Build history of the part. All positions in model axes, mm. Face numbers are marked on the shaded views. A direction names the side the tool comes from. Give positions to 0.01 mm unless a question says otherwise; leave off trailing zeros. Loops run counter-clockwise (first coordinate to the right, second up) from the corner with the lowest first, then second, coordinate; pieces in that order, holes last. Notation, with made-up numbers: (7.5, 41.25) - (54.5, 41.25) arc R25 ccw to (54.5, 53.25) - close; hole circle Ø7 at (-16.75, 47). An arc over 180 degrees is marked (long way). Return JSON: item names as keys, results as strings. Group by question number.
1) Drop flat-ended pins along their axis: pin 1 (5 mm diameter, centred on x = 1, y = 46.5, fed in from +Z); pin 2 (11.5 mm diameter, centred on y = 0, z = 38.1, fed in from -X). Give the stop position or say it passes through.
2) Slice it at A-A (z = 57). List the corners of the cut face in (x, y).
3) Mould opens along Y. For the marked faces 1, 2, 3 and 4 say: released by +Y, released by -Y, zero draft, split by the parting line, or undercut.
4) Slice it at D-D (y = 0). List the corners of the cut face in (x, z) (3 decimals), and give its area (3 significant figures).
5) 3-axis set-ups, long thin cutter, end or side, ignore diameter. For the marked faces 5 and 6: which of +Z, -Z, +X, -X, +Y, -Y reach the whole face in a straight line?
6) Drill centre lines: probe 1 along X at (y, z) = (10, 58); probe 2 along Y at (x, z) = (-71, 38); probe 3 along Y at (x, z) = (-35, 23.5). Where is each one in solid material? Low to high. Write a range as from..to.
7) Slice it at B-B (y = -12.5). List the corners of the cut face in (x, z).
8) Slice it at C-C (x = 0). List the corners of the cut face in (y, z), and give its area (3 significant figures).
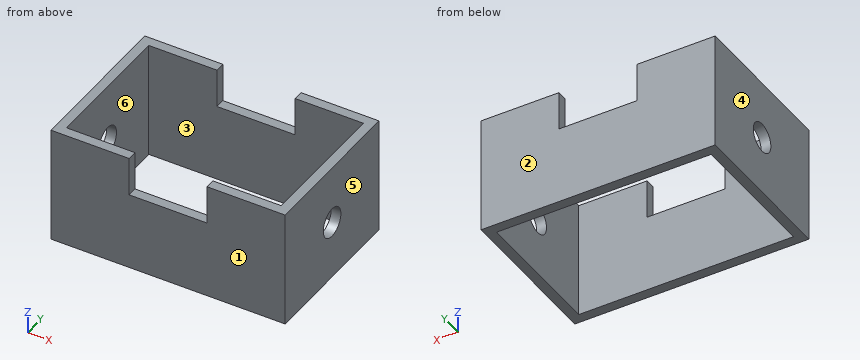
```python
from build123d import *

# Parameters (mm, degrees)
F0_W     = 152.4
F0_H     = 101.6
F0_W_2   = 139.7
F0_H_2   = 88.9
F1_DEPTH = 76.2
F2_W     = 50.8
F2_H     = 25.4
F3_DEPTH = 101.601
F4_R     = 9.525
F5_DEPTH = 152.401


with BuildPart() as f1:
    # F0 (on Top) → F1 (new body)
    with BuildSketch(Plane.XY):
        Rectangle(F0_W, F0_H)
        Rectangle(F0_W_2, F0_H_2, mode=Mode.SUBTRACT)
    extrude(amount=F1_DEPTH)

    # F2 (on face) → F3 (cut, through all)
    with BuildSketch(Plane.XZ.offset(50.8)):
        with Locations((0, 63.5)):
            Rectangle(F2_W, F2_H)
    extrude(amount=-F3_DEPTH, mode=Mode.SUBTRACT)

    # F4 (on face) → F5 (cut, through all)
    with BuildSketch(Plane.YZ.offset(76.2)):
        with Locations((0, 38.1)):
            Circle(F4_R)
    extrude(amount=-F5_DEPTH, mode=Mode.SUBTRACT)


solid = f1.part
```
Results:
{
 "1": {"pin 1": "z = 50.8", "pin 2": "through"},
 "2": {"outline": "(-76.2, -50.8) - (-25.4, -50.8) - (-25.4, -44.45) - (-69.85, -44.45) - (-69.85, 44.45) - (-25.4, 44.45) - (-25.4, 50.8) - (-76.2, 50.8) - close; (25.4, -50.8) - (76.2, -50.8) - (76.2, 50.8) - (25.4, 50.8) - (25.4, 44.45) - (69.85, 44.45) - (69.85, -44.45) - (25.4, -44.45) - close"},
 "3": {"face 1": "released by -Y", "face 2": "released by +Y", "face 3": "undercut", "face 4": "zero draft"},
 "4": {"outline": "(-76.2, 0) - (-69.85, 0) - (-69.85, 28.575) - (-76.2, 28.575) - close; (-76.2, 47.625) - (-69.85, 47.625) - (-69.85, 76.2) - (-76.2, 76.2) - close; (69.85, 0) - (76.2, 0) - (76.2, 28.575) - (69.85, 28.575) - close; (69.85, 47.625) - (76.2, 47.625) - (76.2, 76.2) - (69.85, 76.2) - close", "area": "726 mm2"},
 "5": {"face 5": "+Z, -Z, +X, +Y, -Y", "face 6": "+Z, -Z"},
 "6": {"probe 1": "-76.2..-69.85, 69.85..76.2", "probe 2": "-50.8..-9.52, 9.52..50.8", "probe 3": "-50.8..-44.45, 44.45..50.8"},
 "7": {"outline": "(-76.2, 0) - (-69.85, 0) - (-69.85, 76.2) - (-76.2, 76.2) - close; (69.85, 0) - (76.2, 0) - (76.2, 76.2) - (69.85, 76.2) - close"},
 "8": {"outline": "(-50.8, 0) - (-44.45, 0) - (-44.45, 50.8) - (-50.8, 50.8) - close; (44.45, 0) - (50.8, 0) - (50.8, 50.8) - (44.45, 50.8) - close", "area": "645 mm2"}
}
